Part print with two shaded views. Sizes in mm from the minimum x, y, z corner. Round coordinates to 2 decimals unless told otherwise and drop trailing zeros. Loops run counter-clockwise (first coordinate to the right, second up) from the corner with the lowest first, then second, coordinate; pieces in that order, holes last.
(1) Probe probe 1 along Y at (x, z) = (34, 1.8); probe 2 along X at (y, z) = (34.5, 3.45); probe 3 along X at (y, z) = (22, 4.45) (1 decimal). List the from-to ranges inside material, lowest first.
(2) Mould opens along X. For the marked faces 1, 2 and 3 say: +X half, -X half, draft (parallel to the pull), parting line (faces both ways), or undercut.
(3) Cut at A-A on x = 34. List the corners of the cut face in (y, z), then the cut area to 3 significant figures.
(4) Cut at C-C on z = 3.05. List the corners of the cut face in (x, y).
(5) Cut at D-D on y = 23. List the corners of the cut face in (x, z), then the cut area to 3 significant figures.
(6) Cut at B-B on y = 34. List the corners of the cut face in (x, z), then the cut area to 3 significant figures.
(7) Flat gauge pins, fed straight in: pin 1 (2.5 mm diameter, centred on x = 34, y = 56, fed in from -Z); pin 2 (17 mm diameter, centred on x = 34, y = 34, fed in from +Z); pin 3 (2 mm diameter, centred on x = 47, z = 2.5, fed in from +Y); pin 4 (1 mm diameter, centred on x = 54, z = 2.5, fed in from +Y). Where does each tip first touch, or does it go through?
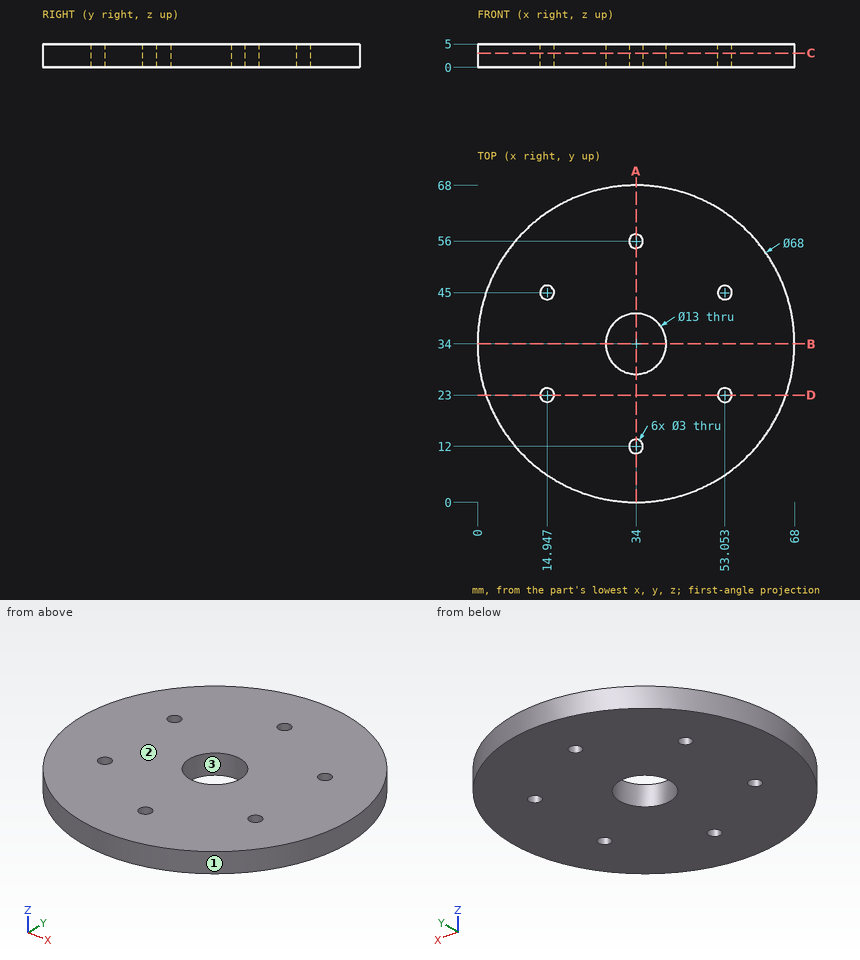
Final values:
1. probe 1: y = 0 to 10.5, 13.5 to 27.5, 40.5 to 54.5, 57.5 to 68
1. probe 2: x = 0 to 27.52, 40.48 to 68
1. probe 3: x = 2.2 to 13.8, 16.1 to 51.9, 54.2 to 65.8
2. face 1: parting line
2. face 2: draft
2. face 3: undercut
3. outline: (0, 0) - (10.5, 0) - (10.5, 5) - (0, 5) - close; (13.5, 0) - (27.5, 0) - (27.5, 5) - (13.5, 5) - close; (40.5, 0) - (54.5, 0) - (54.5, 5) - (40.5, 5) - close; (57.5, 0) - (68, 0) - (68, 5) - (57.5, 5) - close
3. area: 245 mm2
4. outline: circle Ø68 at (34, 34); hole circle Ø3 at (14.95, 23); hole circle Ø3 at (14.95, 45); hole circle Ø13 at (34, 34); hole circle Ø3 at (34, 12); hole circle Ø3 at (34, 56); hole circle Ø3 at (53.05, 23); hole circle Ø3 at (53.05, 45)
5. outline: (1.83, 0) - (13.45, 0) - (13.45, 5) - (1.83, 5) - close; (16.45, 0) - (51.55, 0) - (51.55, 5) - (16.45, 5) - close; (54.55, 0) - (66.17, 0) - (66.17, 5) - (54.55, 5) - close
5. area: 292 mm2
6. outline: (0, 0) - (27.5, 0) - (27.5, 5) - (0, 5) - close; (40.5, 0) - (68, 0) - (68, 5) - (40.5, 5) - close
6. area: 275 mm2
7. pin 1: passes through
7. pin 2: stops at z = 5
7. pin 3: stops at y = 65.81
7. pin 4: stops at y = 61.85
